Geometry: final body of the model. Coordinates: model frame, mm. A direction names the side the tool comes from. Give positions to 0.01 mm unless a question says otherwise; leave off trailing zeros. Loops run counter-clockwise (first coordinate to the right, second up) from the corner with the lowest first, then second, coordinate; pieces in that order, holes last.
1. Section A-A, the plane y = 43. Output: boundary loops of the cut face in (x, z).
2. First-contact query: P1, Ø22, axis at y = 70, z = -146, coming from the -X side; P2, Ø6, axis at x = -58, y = 60.5, coming from the +Z side; P3, Ø6, axis at x = -157, y = 68.5, coming from the -Z side. Flat tips, straight axial feed; report the tip coordinate or a pass-through.
3. Material intervals for line 1 along X through (y, z) = (222.5, 0); line 2 along Y through (x, z) = (16, 213); line 3 along Z through (x, y) = (-57.5, 149.5), sorted ascending.
4. Section D-D, the plane y = 204. Output: boundary loops of the cut face in (x, z).
5. Section C-C, the plane z = 0. Output: boundary loops of the cut face in (x, y).
6. Section B-B, the plane x = 0. Output: boundary loops of the cut face in (y, z), then the cut area to 3 significant figures.
7. Access query for faces 1 (the face through (-184.964, 34.65, -185.742)), 2 (the face through (150, 80, -129)), 3 (the face through (-185.742, 34.65, 184.964)), 4 (the face through (-134.67, 69.86, -176.15)), 5 (the face through (39.048, 166.205, 123.997)). Directions: +Z, -Z, +X, -X, +Y, -Y. A direction counts if a zero-diameter tool reaches every point of the face in a straight line with its end or side. Return the directions, or none.
8. Draft query along X for faces 6 (the face through (-129, 80, -150)), 7 (the face through (275.14, 3.94, -36.12)), 8 (the face through (119.689, 70, 150)), 9 (the face through (176.348, 69.86, -164.985)). Return one class per face: +X half, -X half, draft (parallel to the pull), parting line (faces both ways), or undercut.
from build123d import *

# Parameters (mm, degrees)
SKETCH1_R                = 277.5
BOSS_EXTRUDE1_DEPTH      = 10
SKETCH2_W                = 400
SKETCH2_H                = 400
BOSS_EXTRUDE2_DEPTH      = 50
FILLET1_R                = 50
SKETCH3_R                = 130
BOSS_EXTRUDE3_DEPTH      = 200
SKETCH4_R                = 160
BOSS_EXTRUDE4_DEPTH      = 20
SKETCH7_R                = 100
CUT_EXTRUDE2_DEPTH       = 200
FILLET3_R                = 15
FILLET4_R                = 2
BOSS_EXTRUDE6_DEPTH      = 20
SKETCH9_R                = 20
CUT_EXTRUDE3_DEPTH       = 6
FILLET5_R                = 12
FILLET6_R                = 6
CIRPATTERN1_COUNT        = 4
FILLET5_OF_CIRPATTERN1_R = 12
FILLET6_OF_CIRPATTERN1_R = 6


with BuildPart() as part:
    # Sketch1 → Boss-Extrude1 (new body)
    with BuildSketch(Plane(origin=(0, 0, 0), x_dir=(1, 0, 0), z_dir=(0, 1, 0))):
        with Locations(Location((0, 0, 0), (0, 0, 270))):
            Circle(SKETCH1_R)
    extrude(amount=BOSS_EXTRUDE1_DEPTH)

    # Sketch2 → Boss-Extrude2 (add)
    with BuildSketch(Plane(origin=(0, 10, 0), x_dir=(1, 0, 0), z_dir=(0, 1, 0))):
        Rectangle(SKETCH2_W, SKETCH2_H)
    extrude(amount=BOSS_EXTRUDE2_DEPTH)

    # Fillet1
    # the kernel refuses this fillet: 50 mm, written as the material it takes off along each edge
    with BuildSketch(Plane(origin=(-200, 10, -200), x_dir=(0, 0, 1), z_dir=(0, 1, 0)), Plane(origin=(-200, 10, 200), x_dir=(1, 0, 0), z_dir=(0, 1, 0)), Plane(origin=(200, 10, -200), x_dir=(-1, 0, 0), z_dir=(0, 1, 0))) as fillet1_piece_1:
        with BuildLine():
            CenterArc((FILLET1_R, FILLET1_R), FILLET1_R, 180, 90)
            Line((0, FILLET1_R), (0, 0))
            Line((0, 0), (FILLET1_R, 0))
        make_face()
    extrude(amount=175, mode=Mode.SUBTRACT)
    with BuildSketch(Plane(origin=(200, 10, 200), x_dir=(-1, 0, 0), z_dir=(0, 1, 0))) as fillet1_piece_2:
        with BuildLine():
            CenterArc((FILLET1_R, -FILLET1_R), FILLET1_R, 90, 90)
            Line((0, -FILLET1_R), (0, 0))
            Line((0, 0), (FILLET1_R, 0))
        make_face()
    extrude(amount=175, mode=Mode.SUBTRACT)

    # Sketch3 → Boss-Extrude3 (add)
    with BuildSketch(Plane(origin=(0, 60, 0), x_dir=(1, 0, 0), z_dir=(0, 1, 0))):
        with Locations(Location((0, 0, 0), (0, 0, 270))):
            Circle(SKETCH3_R)
    extrude(amount=BOSS_EXTRUDE3_DEPTH)

    # Sketch4 → Boss-Extrude4 (add)
    with BuildSketch(Plane(origin=(0, 260, 0), x_dir=(1, 0, 0), z_dir=(0, 1, 0))):
        with Locations(Location((0, 0, 0), (0, 0, 270))):
            Circle(SKETCH4_R)
    extrude(amount=BOSS_EXTRUDE4_DEPTH)

    # Sketch7 → Cut-Extrude2 (cut)
    with BuildSketch(Plane(origin=(0, 280, 0), x_dir=(1, 0, 0), z_dir=(0, 1, 0))):
        with Locations(Location((0, 0, 0), (0, 0, 270))):
            Circle(SKETCH7_R)
    extrude(amount=-CUT_EXTRUDE2_DEPTH, mode=Mode.SUBTRACT)

    # Fillet3
    fillet3_edges = [part.edges().sort_by_distance(p)[0] for p in [
        (0, 60, -130),
    ]]
    fillet(fillet3_edges, radius=FILLET3_R)

    # Fillet4
    fillet4_edges = [part.edges().sort_by_distance(p)[0] for p in [
        (0, 10, -277.5),
        (0, 280, -160),
    ]]
    fillet(fillet4_edges, radius=FILLET4_R)

    # Sketch8 → Boss-Extrude6 (add)
    with BuildSketch(Plane(origin=(0, 60, 0), x_dir=(1, 0, 0), z_dir=(0, 1, 0))):
        Polygon((150, -185), (180.310889132, -167.5), (180.310889132, -132.5), (150, -115), (119.689110868, -132.5), (119.689110868, -167.5), align=None)
    boss_extrude6 = extrude(amount=BOSS_EXTRUDE6_DEPTH)

    # Sketch9 → Cut-Extrude3 (cut)
    with BuildSketch(Plane(origin=(0, 80, 0), x_dir=(1, 0, 0), z_dir=(0, 1, 0))):
        with Locations(Location((150, -150, 0), (0, 0, 270))):
            Circle(SKETCH9_R)
    cut_extrude3 = extrude(amount=-CUT_EXTRUDE3_DEPTH, mode=Mode.SUBTRACT)

    # Fillet5
    # the kernel refuses this fillet: 12 mm, written as the material it adds along each edge
    with BuildSketch(Plane(origin=(150, 74, 150), x_dir=(0, 0, 1), z_dir=(-1, 0, 0))) as fillet5_piece_1:
        with BuildLine():
            CenterArc((9.607695155, 12), FILLET5_R, 270, 60)
            Line((9.607695155, 0), (9.607695155, -0.24))
            Line((9.607695155, -0.24), (20, -0.24))
            Line((20, -0.24), (20.24, 0))
            ThreePointArc((20.24, 0), (20.24, 3), (20.207846097, 5.88))
            Line((20.207846097, 5.88), (20, 6))
        make_face()
    revolve(axis=Axis((150, 74, 150), (0, 1, 0)))

    # Fillet6
    fillet6_edges = [part.edges().sort_by_distance(p)[0] for p in [
        (119.689110868, 70, 167.5),
        (150, 70, 185),
        (180.310889132, 70, 167.5),
        (180.310889132, 70, 132.5),
        (150, 70, 115),
        (119.689110868, 70, 132.5),
    ]]
    fillet(fillet6_edges, radius=FILLET6_R)

    # CirPattern1: Boss-Extrude6, Cut-Extrude3 ×4 about axis
    cirpattern1_axis = Axis((0, 0, 0), (0, 1, 0))
    add([boss_extrude6.rotate(cirpattern1_axis, i * 360 / CIRPATTERN1_COUNT) for i in range(1, CIRPATTERN1_COUNT)])
    add([cut_extrude3.rotate(cirpattern1_axis, i * 360 / CIRPATTERN1_COUNT) for i in range(1, CIRPATTERN1_COUNT)], mode=Mode.SUBTRACT)

    # Fillet5 of CirPattern1
    # the kernel refuses this fillet: 12 mm, written as the material it adds along each edge
    with BuildSketch(Plane(origin=(150, 74, -150), x_dir=(1, 0, 0), z_dir=(0, 0, 1))) as fillet5_of_cirpattern1_piece_1:
        with BuildLine():
            CenterArc((9.607695155, 12), FILLET5_OF_CIRPATTERN1_R, 270, 60)
            Line((9.607695155, 0), (9.607695155, -0.24))
            Line((9.607695155, -0.24), (20, -0.24))
            Line((20, -0.24), (20.24, 0))
            ThreePointArc((20.24, 0), (20.24, 3), (20.207846097, 5.88))
            Line((20.207846097, 5.88), (20, 6))
        make_face()
    revolve(axis=Axis((150, 74, -150), (0, 1, 0)))
    with BuildSketch(Plane(origin=(-150, 74, -150), x_dir=(0, 0, -1), z_dir=(1, 0, 0))) as fillet5_of_cirpattern1_piece_2:
        with BuildLine():
            CenterArc((9.607695155, 12), FILLET5_OF_CIRPATTERN1_R, 270, 60)
            Line((9.607695155, 0), (9.607695155, -0.24))
            Line((9.607695155, -0.24), (20, -0.24))
            Line((20, -0.24), (20.24, 0))
            ThreePointArc((20.24, 0), (20.24, 3), (20.207846097, 5.88))
            Line((20.207846097, 5.88), (20, 6))
        make_face()
    revolve(axis=Axis((-150, 74, -150), (0, 1, 0)))
    with BuildSketch(Plane(origin=(-150, 74, 150), x_dir=(-1, 0, 0), z_dir=(0, 0, -1))) as fillet5_of_cirpattern1_piece_3:
        with BuildLine():
            CenterArc((9.607695155, 12), FILLET5_OF_CIRPATTERN1_R, 270, 60)
            Line((9.607695155, 0), (9.607695155, -0.24))
            Line((9.607695155, -0.24), (20, -0.24))
            Line((20, -0.24), (20.24, 0))
            ThreePointArc((20.24, 0), (20.24, 3), (20.207846097, 5.88))
            Line((20.207846097, 5.88), (20, 6))
        make_face()
    revolve(axis=Axis((-150, 74, 150), (0, 1, 0)))

    # Fillet6 of CirPattern1
    fillet6_of_cirpattern1_edges = [part.edges().sort_by_distance(p)[0] for p in [
        (167.5, 70, -119.689110868),
        (185, 70, -150),
        (167.5, 70, -180.310889132),
        (132.5, 70, -180.310889132),
        (115, 70, -150),
        (132.5, 70, -119.689110868),
        (-119.689110868, 70, -167.5),
        (-150, 70, -185),
        (-180.310889132, 70, -167.5),
        (-180.310889132, 70, -132.5),
        (-150, 70, -115),
        (-119.689110868, 70, -132.5),
        (-167.5, 70, 119.689110868),
        (-185, 70, 150),
        (-167.5, 70, 180.310889132),
        (-132.5, 70, 180.310889132),
        (-115, 70, 150),
        (-132.5, 70, 119.689110868),
    ]]
    fillet(fillet6_of_cirpattern1_edges, radius=FILLET6_OF_CIRPATTERN1_R)


solid = part.part
Answers below:
1. outline: (-200, -150) arc R50 ccw to (-150, -200) - (150, -200) arc R50 ccw to (200, -150) - (200, 150) arc R50 ccw to (150, 200) - (-150, 200) arc R50 ccw to (-200, 150) - close
2. P1: stops at x = -200
2. P2: stops at z = 200
2. P3: stops at z = -182.69
3. line 1: x = -130 to -100, 100 to 130
3. line 2: y = 0 to 10
3. line 3: z = -116.59 to -81.82, 81.82 to 116.59
4. outline: circle Ø260 at (0, 0); hole circle Ø200 at (0, 0)
5. outline: (-277.5, 0) - (277.5, 0) - (277.5, 8) arc R2 ccw to (275.5, 10) - (200, 10) - (200, 60) - (145, 60) arc R15 cw to (130, 75) - (130, 260) - (160, 260) - (160, 278) arc R2 ccw to (158, 280) - (100, 280) - (100, 80) - (-100, 80) - (-100, 280) - (-158, 280) arc R2 ccw to (-160, 278) - (-160, 260) - (-130, 260) - (-130, 75) arc R15 cw to (-145, 60) - (-200, 60) - (-200, 10) - (-275.5, 10) arc R2 ccw to (-277.5, 8) - close
6. outline: (0, -277.5) - (8, -277.5) arc R2 ccw to (10, -275.5) - (10, -200) - (60, -200) - (60, -145) arc R15 cw to (75, -130) - (260, -130) - (260, -160) - (278, -160) arc R2 ccw to (280, -158) - (280, -100) - (80, -100) - (80, 100) - (280, 100) - (280, 158) arc R2 ccw to (278, 160) - (260, 160) - (260, 130) - (75, 130) arc R15 cw to (60, 145) - (60, 200) - (10, 200) - (10, 275.5) arc R2 ccw to (8, 277.5) - (0, 277.5) - close
6. area: 44,000 mm2
7. face 1: -Z, -X, +Y
7. face 2: -Z, +X, +Y
7. face 3: +Z, -X, +Y
7. face 4: -Z, +Y
7. face 5: none
8. face 6: draft
8. face 7: parting line
8. face 8: undercut
8. face 9: +X half
